Work out the finished part from the listing and answer in its coordinate system (mm). Face numbers are marked on the shaded views. Coordinates: 2 decimals unless noted, no trailing zeros. Order: outer loops, then holes, each group sorted by start corner. A loop starts at its lowest first (then second) coordinate and runs counter-clockwise, first axis right, second up. Notation, with made-up numbers: (46.5, 64) -> (68.5, 64) arc R17 cw to (68.5, 86) -> close; hole circle Ø10 at (83.5, 58). An arc over 180 degrees is marked (long way). Answer as CSV lines item,"result". Start each with the question number.
Item 1: Each of these flat-tipped pins is pushed along its axis until it touches: pin 1 Ø3 at (x, y) = (-10.5, 61) entering from +Z; pin 2 Ø12 at (x, y) = (-10.5, 44.5) entering from -Z; pin 3 Ø4 at (y, z) = (38.5, -7) entering from +X. Where does it stop, or does it pass through?
Item 2: Section B-B (y = 74.5) is taken. Write down the section's boundary in (x, z).
Item 3: Straight lines are drawn through the part: L1, parallel to Z at x = -6, y = 87; L2, parallel to Z at x = 1, y = 66.5; L3, parallel to Z at x = -9.5, y = 89. For each, find the intervals that lie inside material, in ascending order.
Item 4: For a pull along X with two mould halves and no side action, classify the marked faces 1, 2 and 3 as pulls with the +X half, pulls with the -X half, needs draft (parallel to the pull), parting line crosses it, or undercut.
Item 5: Section A-A (y = 36) is taken. Write down the section's boundary in (x, z), then the cut area to 3 significant figures.
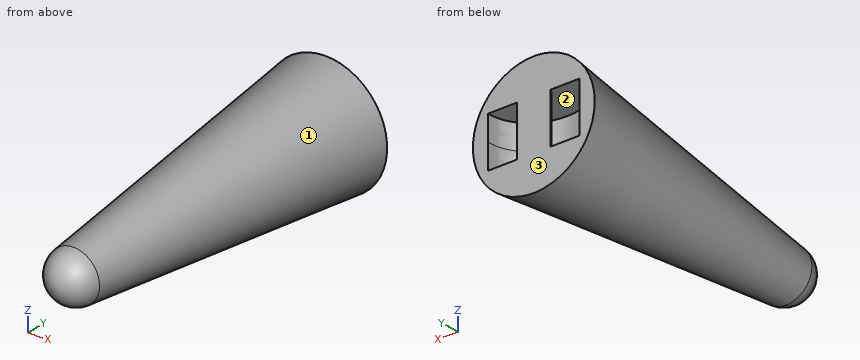
```python
from build123d import *

# Parameters (mm, degrees)
ENL_V_MAT_EXTRU_1_DEPTH      = 7.5
ENL_V_MAT_EXTRU_1_DEPTH_BACK = 7.5
BOSS_EXTRU_1_REACH           = 27.5
ECHELLE1_SCALE               = 0.8


with BuildPart() as part:
    # Esquisse1 → R_volution1 (revolve)
    with BuildSketch(Plane.XY):
        with BuildLine():
            Line((0, 0), (0, 100))
            Line((0, 100), (-18, 100))
            Line((-18, 100), (-7.593007693, 6.792401612))
            ThreePointArc((-7.593007693, 6.792401612), (-5.093880777, 1.945904787), (0, 0))
        make_face()
    revolve(axis=Axis((0, 0, 0), (0, 1, 0)))

    # Esquisse2 → Enl_v. mat.-Extru.1 (cut, two sides)
    with BuildSketch(Plane.XY) as enl_v_mat_extru_1_sk:
        with BuildLine():
            Line((-13.5, 100), (13.5, 100))
            add(Edge.make_bspline(
                [(-13.5, 100), (-13.291113541, 83.520875666), (13.291113541, 83.520875666), (13.5, 100)],
                knots=[0, 0, 0, 0, 1, 1, 1, 1], degree=3))
        make_face()
    extrude(amount=ENL_V_MAT_EXTRU_1_DEPTH, mode=Mode.SUBTRACT)
    extrude(enl_v_mat_extru_1_sk.sketch, amount=-ENL_V_MAT_EXTRU_1_DEPTH_BACK, mode=Mode.SUBTRACT)

    # Esquisse3 → Boss.-Extru.1 (add, up to next)
    with BuildSketch(Plane.XY.offset(-7.5), mode=Mode.PRIVATE) as boss_extru_1_sk1:
        with BuildLine():
            Line((-5, 100), (5, 100))
            add(Edge.make_bspline(
                [(-5, 100), (0, 91.498247822), (5, 100)],
                knots=[0, 0, 0, 1, 1, 1], degree=2))
        make_face()
    boss_extru_1_tool1 = extrude(boss_extru_1_sk1.sketch, amount=BOSS_EXTRU_1_REACH, mode=Mode.PRIVATE) - part.part
    add(boss_extru_1_tool1.solids().sort_by_distance((0, 98.29965, -7.5))[0])


with BuildPart() as part_1:
    # Echelle1: scaled about (-4e-09, 62.219241992, 3e-09)
    add(part.part.scale(ECHELLE1_SCALE).moved(Location((-1e-09, 12.443848398, 1e-09))))


solid = part_1.part
```
Checked values:
1,pin 1,"stops at z = 6.15"
1,pin 2,"stops at z = -7.93"
1,pin 3,"stops at x = 6.75"
2,outline,"circle Ø24.79 at (0, 0)"
3,L1,"z = -12.42 to -6, 6 to 12.42"
3,L2,"z = -11.46 to 11.46"
3,L3,"z = -10.3 to -6, 6 to 10.3"
4,face 1,"parting line crosses it"
4,face 2,"undercut"
4,face 3,"needs draft"
5,outline,"circle Ø16.2 at (0, 0)"
5,area,"206 mm^2"
